from build123d import *

# Parameters (mm, degrees)
F0_R     = 5.2549557128
F1_DEPTH = 11.43
F1_TAPER = 15
F0_R_2   = 3.9878
F0_R_3   = 4.0731099985
F3_DEPTH = 0.254


with BuildPart() as f1:
    # F0 (on Top) → F1 (new body)
    with BuildSketch(Plane.XY):
        Circle(F0_R)
    extrude(amount=F1_DEPTH, taper=F1_TAPER)



with BuildPart() as f1b:
    # F0 (on Top) → F1, piece 2 (new body)
    with BuildSketch(Plane.XY):
        with Locations((31.517803368, 0)):
            Circle(F0_R_2)
    extrude(amount=F1_DEPTH, taper=F1_TAPER)


with BuildPart() as f1c:
    # F0 (on Top) → F1, piece 3 (new body)
    with BuildSketch(Plane.XY):
        with Locations((-31.517803368, 0)):
            Circle(F0_R_3)
    extrude(amount=F1_DEPTH, taper=F1_TAPER)


with BuildPart() as f1_1:
    add(f1.part)

    add(f1b.part)  # F3 merges F1b

    add(f1c.part)  # F3 merges F1c
    # F2 (on Front) → F3 (join)
    with BuildSketch(Plane.XZ):
        Polygon((-31.5407924354, 2.1590758115), (-31.0882329941, 0), (0, 0), (32.4205830693, 0), (32.4205830693, 2.1590758115), (0, 2.1590758115), align=None)
    extrude(amount=-F3_DEPTH)


solid = f1_1.part
Could you check a few things on this model? Use its own coordinates, in mm. Coordinates: 2 decimals unless noted, no trailing zeros. Order: outer loops, then holes, each group sorted by start corner. A loop starts at its lowest first (then second) coordinate and runs counter-clockwise, first axis right, second up.
Q1. Suppose I cut it at A-A on x = -11. Please give me the cut outline in (y, z), and give its area (3 significant figures).
Q2. Will these pins go through, and if not, where does the flat tip stop? pin 1 (0.6 mm diameter, centred on x = 17, z = 1, fed in from +Y); pin 2 (2.5 mm diameter, centred on x = 19.5, z = 1.5, fed in from -Y); pin 3 (2 mm diameter, centred on y = 3.5, z = 3, fed in from +X).
Q3. Suppose I cut it at D-D on x = 0. Please give me the cut outline in (y, z).
Q4. Suppose I cut it at C-C on y = -3. Give the number of separate pieces and of enclosed holes in the cut face, and give its area (3 significant figures).
Q5. Thinking about a two-plate mould opening in X: for faces 1 (the flat face through (32, 0, 11.43)), 2 (the flat face through (-17, 0, 1)), which applies, released by +X, released by -X, zero draft, split by the parting line, or undercut?
Q6. Suppose I cut it at B-B on z = 10.5. Please give me the cut outline in (x, y), and give its area (3 significant figures).
Q7. Please list where these lines run through material, in increasing order: L1, parallel to X at y = -0.75, z = 2.25; L2, parallel to X at y = 0.75, z = 0.5; L3, parallel to Y at x = 32, z = 2.25.
Answer:
1. outline: (0, 0) - (0.25, 0) - (0.25, 2.16) - (0, 2.16) - close
1. area: 0.548 mm2
2. pin 1: stops at y = 0.25
2. pin 2: stops at y = 0
2. pin 3: stops at x = 33.56
3. outline: (-5.25, 0) - (5.25, 0) - (2.19, 11.43) - (-2.19, 11.43) - close
4. separate pieces: 3
4. enclosed holes: 0
4. area: 72.4 mm2
5. face 1: zero draft
5. face 2: undercut
6. outline: circle Ø2.52 at (-31.52, 0); circle Ø4.88 at (0, 0); circle Ø2.35 at (31.52, 0)
6. area: 28.0 mm2
7. L1: x = -34.91 to -28.13, -4.59 to 4.59, 28.22 to 34.82
7. L2: x = -35.38 to -27.65, -5.07 to 5.07, 27.74 to 35.3
7. L3: y = -3.35 to 3.35
